from build123d import *

# Parameters (mm, degrees)
F1_DEPTH = 1100
F3_DEPTH = 19.001
F4_W     = 27
F4_H     = 5.5
F4_W_2   = 10
F5_DEPTH = 1051.4265870314


with BuildPart() as f1:
    # F0 (on Top) → F1 (new body)
    with BuildSketch(Plane.XY):
        Polygon((0, -4), (0, -9.5), (136, -9.5), (136, -4), (146, -4), (146, 4), (116, 4), (110.5, 9.5), (0, 9.5), (0, 4), (12, 4), (12, -4), align=None)
    extrude(amount=F1_DEPTH)

    # F2 (on face) → F3 (cut, through all)
    with BuildSketch(Plane(origin=(0, 9.5, 0), x_dir=(-1, 0, 0), z_dir=(0, 1, 0))):
        Polygon((-110.5, 1100), (-608.1546681334, 1100), (-110.5, 1047.6943866794), align=None)
        Polygon((0, 1100), (0, 1036.0803686826), (819, 950), (819, 1100), align=None)
        Polygon((-110.5, 1100), (-110.5, 1047.6943866794), (0, 1036.0803686826), (0, 1100), align=None)
    extrude(amount=-F3_DEPTH, mode=Mode.SUBTRACT)

    # F4 (on face) → F5 (cut, through all)
    with BuildSketch(Plane(origin=(0, 0, 0), x_dir=(1, 0, 0), z_dir=(0, 0, -1))):
        with Locations((132.5, -6.75)):
            Rectangle(F4_W, F4_H)
        Polygon((136, 9.5), (119, 9.5), (119, -4), (146, -4), (146, 4), (136, 4), align=None)
        with Locations((141, 6.75)):
            Rectangle(F4_W_2, F4_H)
    extrude(amount=-F5_DEPTH, mode=Mode.SUBTRACT)


solid = f1.part
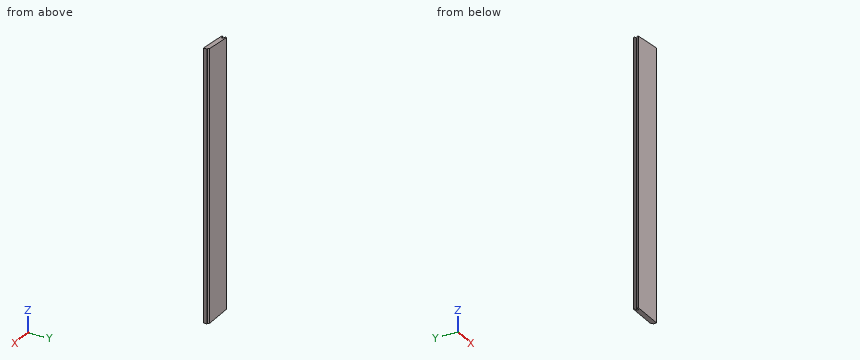
Source: CAD feature listing. Evaluate the final solid. Frame: model axes, mm. Give positions to 0.01 mm unless a question says otherwise; leave off trailing zeros. Write each loop counter-clockwise with the first axis right and the second up, starting at its lowest first coordinate (ties: lowest second). Pieces come first, ordered by that corner, then holes. Notation, with made-up numbers: (87, 13.5) -> (131, 13.5) arc R28 ccw to (131, 51.5) -> close; hole circle Ø4 at (-32, -10). An arc over 180 degrees is marked (long way). Return JSON: item names as keys, results as strings. Group by question number.
1. Material intervals for line 1 (X direction, y = 1.25, z = 488); line 2 (X direction, y = 4.5, z = 174); line 3 (Z direction, x = 19, y = -8), sorted ascending. Write a range as from..to.
2. Section A-A, the plane z = 862. Output: boundary loops of the cut face in (x, y), then the cut area to 3 significant figures.
3. Pin query (flat end, axial travel): pin 1 Ø4 at (x, y) = (64.5, -1.5) entering from +Z; pin 2 Ø2.5 at (x, z) = (117.5, 756) entering from +Y; pin 3 Ø6 at (x, y) = (81, 6) entering from +Z. Return the tip coordinate at first contact, or that it passes through.
4. Section B-B, the plane y = -0.25. Output: boundary loops of the cut face in (x, z).
Determined:
{
 "1": {"line 1": "x = 12..119", "line 2": "x = 0..115.5", "line 3": "z = 0..1038.08"},
 "2": {"outline": "(0, -9.5) -> (119, -9.5) -> (119, 4) -> (116, 4) -> (110.5, 9.5) -> (0, 9.5) -> (0, 4) -> (12, 4) -> (12, -4) -> (0, -4) -> close", "area": "2,130 mm2"},
 "3": {"pin 1": "stops at z = 1043.07", "pin 2": "stops at y = 4", "pin 3": "stops at z = 1044.91"},
 "4": {"outline": "(12, 0) -> (119, 0) -> (119, 1048.59) -> (12, 1037.34) -> close"}
}
